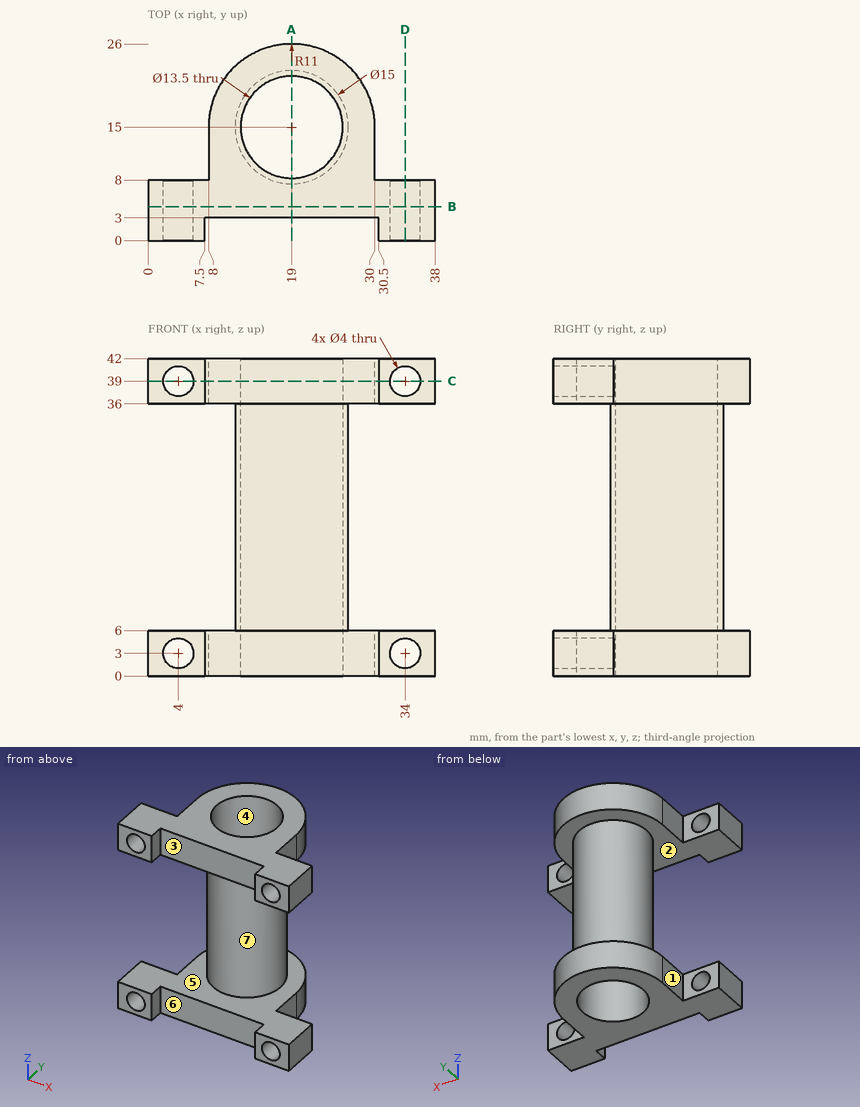
The drawing under review shows one solid part. Ordinate dimensions are in mm from its lowest x, y, z. A direction names the side the tool comes from. Round coordinates to 2 decimals unless told otherwise and drop trailing zeros. Loops run counter-clockwise (first coordinate to the right, second up) from the corner with the lowest first, then second, coordinate; pieces in that order, holes last. Notation, with made-up numbers: (59.5, -3) - (85.5, -3) arc R12 ccw to (85.5, 2) - close; hole circle Ø3 at (-21, -26). An arc over 180 degrees is marked (long way). Use one line per item in the form item = value.
Item 1: Tool access review of the marked faces 1, 2 and 3: name each direction out of +Z, -Z, +X, -X, +Y, -Y from which nothing blocks a thin tool from reaching the whole face with its end or side.
Answers:
face_1 = +Z, -Z, -X, +Y
face_2 = none
face_3 = +Z, -Z, -Y
Item 2: For line 1 (X direction, y = 2.25, z = 39); line 2 (X direction, y = 4.75, z = 39); line 3 (Z direction, x = 26.5, y = 17.25), list the stretches that pass through material, from the lowest coordinate up.
Answers:
line_1 = 0 to 2, 6 to 7.5, 30.5 to 32, 36 to 38
line_2 = 0 to 2, 6 to 32, 36 to 38
line_3 = 0 to 6, 36 to 42
Item 3: Consider section B-B on y = 4.5. Write out the cut boundary in (x, z), then the cut area to 3 significant figures.
Answers:
outline = (0, 0) - (38, 0) - (38, 6) - (0, 6) - close; (0, 36) - (38, 36) - (38, 42) - (0, 42) - close; hole circle Ø4 at (4, 3); hole circle Ø4 at (4, 39); hole circle Ø4 at (34, 3); hole circle Ø4 at (34, 39)
area = 406 mm^2
Item 4: Consider section C-C on z = 39. Write out the cut boundary in (x, y).
Answers:
outline = (0, 0) - (2, 0) - (2, 8) - (0, 8) - close; (6, 0) - (7.5, 0) - (7.5, 3) - (30.5, 3) - (30.5, 0) - (32, 0) - (32, 8) - (30, 8) - (30, 15) arc R11 ccw to (8, 15) - (8, 8) - (6, 8) - close; (36, 0) - (38, 0) - (38, 8) - (36, 8) - close; hole circle Ø13.5 at (19, 15)
Item 5: Consider section D-D on x = 34. Write out the cut boundary in (y, z).
Answers:
outline = (0, 0) - (8, 0) - (8, 1) - (0, 1) - close; (0, 5) - (8, 5) - (8, 6) - (0, 6) - close; (0, 36) - (8, 36) - (8, 37) - (0, 37) - close; (0, 41) - (8, 41) - (8, 42) - (0, 42) - close
Item 6: Mouldability with a two-part tool opening along Y and no side actions: class the marked faces 4, 5, 6 and 7 as +Y half, -Y half, draft (parallel to the pull), parting line (faces both ways), or undercut.
Answers:
face_4 = undercut
face_5 = draft
face_6 = -Y half
face_7 = parting line
Item 7: Clearance check with flat-ended pins moving along their axes: P1, Ø5, axis at y = 11, z = 25.5, coming from the +X side; P2, Ø3, axis at x = 3, z = 40, coming from the +Y side; P3, Ø2, axis at y = 20.5, z = 23, coming from the -X side; P4, Ø3.5, axis at y = 1.5, z = 3.5, coming from the -X side. State where each tip first meets the part, or that it passes through.
Answers:
P1 = 26.35
P2 = 8
P3 = 13
P4 = 0
Item 8: Consider section A-A on x = 19. Write out the cut boundary in (y, z), then the cut area to 3 significant figures.
Answers:
outline = (3, 0) - (8.25, 0) - (8.25, 42) - (3, 42) - (3, 36) - (7.5, 36) - (7.5, 6) - (3, 6) - close; (21.75, 0) - (26, 0) - (26, 6) - (22.5, 6) - (22.5, 36) - (26, 36) - (26, 42) - (21.75, 42) - close
area = 159 mm^2
